from build123d import *

# Parameters (mm, degrees)
SKETCH1_W                = 71.12
SKETCH1_H                = 55.88
PCB_BASE_DEPTH           = 2.54
SKETCH1_4_W              = 78.74
SKETCH1_4_H              = 63.5
SKETCH1_4_W_2            = 71.12
SKETCH1_4_H_2            = 55.88
PCB_WALL_DEPTH           = 25.4
SKETCH2_W                = 27.94
SKETCH2_H                = 15.748
PCB_GAP_DEPTH            = 3.81
LID_HOLE_1_DEPTH         = 3.81
HOLE_SLIDE_1_DEPTH       = 2.54
LID_HOLE_2_START         = -3.81
LID_HOLE_2_DEPTH         = 3.81
HOLE_SLIDE_2_START       = -2.54
HOLE_SLIDE_2_DEPTH       = 2.54
SKETCH5_W                = 27.94
SKETCH5_H                = 5.08
BOSS_EXTRUDE3_DEPTH      = 48.768
BOSS_EXTRUDE4_DEPTH      = 8.89
BOSS_EXTRUDE4_DEPTH_BACK = 1.27
SKETCH7_W                = 38.1
SKETCH7_H                = 25.4
BOSS_EXTRUDE5_DEPTH      = 25.4
SKETCH9_W                = 57.658
SKETCH9_H                = 25.4
BOSS_EXTRUDE6_DEPTH      = 3.81


with BuildPart() as part:
    # Sketch1 → pcb-base (new body)
    with BuildSketch(Plane(origin=(0, 0, 0), x_dir=(1, 0, 0), z_dir=(0, 1, 0))):
        Rectangle(SKETCH1_W, SKETCH1_H)
    extrude(amount=PCB_BASE_DEPTH)

    # Sketch1<4> → pcb-wall (add)
    with BuildSketch(Plane(origin=(0, 0, 0), x_dir=(1, 0, 0), z_dir=(0, 1, 0))):
        Rectangle(SKETCH1_4_W, SKETCH1_4_H)
        Rectangle(SKETCH1_4_W_2, SKETCH1_4_H_2, mode=Mode.SUBTRACT)
    extrude(amount=PCB_WALL_DEPTH)

    # Sketch2 → pcb-gap (cut)
    with BuildSketch(Plane.ZY.offset(39.37)):
        with Locations((-12.7, 12.446)):
            Rectangle(SKETCH2_W, SKETCH2_H)
    extrude(amount=-PCB_GAP_DEPTH, mode=Mode.SUBTRACT)

    # Sketch4 → lid-hole-1 (cut)
    with BuildSketch(Plane(origin=(0, 0, 27.94), x_dir=(-1, 0, 0), z_dir=(0, 0, -1))):
        with BuildLine():
            ThreePointArc((3.175, 17.080851973), (0, 18.415), (-3.175, 17.080851973))
            Line((-3.175, 17.080851973), (-3.175, 13.97))
            Line((-3.175, 13.97), (3.175, 13.97))
            Line((3.175, 13.97), (3.175, 17.080851973))
        make_face()
        with BuildLine():
            Line((-3.175, 13.97), (-3.175, 17.080851973))
            ThreePointArc((-3.175, 17.080851973), (-1.680052083, 9.854729657), (4.445, 13.97))
            ThreePointArc((4.445, 13.97), (4.115270343, 15.650052083), (3.175, 17.080851973))
            Line((3.175, 17.080851973), (3.175, 13.97))
            Line((3.175, 13.97), (-3.175, 13.97))
        make_face()
    extrude(amount=-LID_HOLE_1_DEPTH, mode=Mode.SUBTRACT)

    # Sketch4<6> → hole-slide-1 (cut)
    with BuildSketch(Plane(origin=(0, 0, 27.94), x_dir=(-1, 0, 0), z_dir=(0, 0, -1))):
        with BuildLine():
            Line((3.175, 25.4), (-3.175, 25.4))
            Line((-3.175, 25.4), (-3.175, 17.080851973))
            ThreePointArc((-3.175, 17.080851973), (0, 18.415), (3.175, 17.080851973))
            Line((3.175, 17.080851973), (3.175, 25.4))
        make_face()
    extrude(amount=-HOLE_SLIDE_1_DEPTH, mode=Mode.SUBTRACT)

    # Sketch3 → lid-hole-2 (cut)
    with BuildSketch(Plane.XY.offset(-27.94).offset(LID_HOLE_2_START)):
        with BuildLine():
            Line((-3.175, 17.080851973), (-3.175, 13.97))
            Line((-3.175, 13.97), (3.175, 13.97))
            Line((3.175, 13.97), (3.175, 17.080851973))
            ThreePointArc((3.175, 17.080851973), (0, 18.415), (-3.175, 17.080851973))
        make_face()
        with BuildLine():
            Line((3.175, 13.97), (-3.175, 13.97))
            Line((-3.175, 13.97), (-3.175, 17.080851973))
            ThreePointArc((-3.175, 17.080851973), (-1.680052083, 9.854729657), (4.445, 13.97))
            ThreePointArc((4.445, 13.97), (4.115270343, 15.650052083), (3.175, 17.080851973))
            Line((3.175, 17.080851973), (3.175, 13.97))
        make_face()
    extrude(amount=LID_HOLE_2_DEPTH, mode=Mode.SUBTRACT)

    # Sketch3<5> → hole-slide-2 (cut)
    with BuildSketch(Plane.XY.offset(-27.94).offset(HOLE_SLIDE_2_START)):
        with BuildLine():
            Line((-3.175, 25.4), (-3.175, 17.080851973))
            ThreePointArc((-3.175, 17.080851973), (0, 18.415), (3.175, 17.080851973))
            Line((3.175, 17.080851973), (3.175, 25.4))
            Line((3.175, 25.4), (-3.175, 25.4))
        make_face()
    extrude(amount=HOLE_SLIDE_2_DEPTH, mode=Mode.SUBTRACT)

    # Sketch5 → Boss-Extrude3 (add)
    with BuildSketch(Plane.ZY.offset(39.37)):
        Polygon((-31.75, 25.4), (-31.75, 3.81), (-26.67, 3.81), (-26.67, 4.572), (-26.67, 20.32), (-26.67, 25.4), align=None)
        with Locations((-12.7, 22.86)):
            Rectangle(SKETCH5_W, SKETCH5_H)
        Polygon((1.27, 3.81), (6.35, 3.81), (6.35, 25.4), (1.27, 25.4), (1.27, 20.32), (1.27, 4.572), align=None)
        Polygon((-31.75, 3.81), (-31.75, 0), (6.35, 0), (6.35, 3.81), (1.27, 3.81), (-26.67, 3.81), align=None)
    extrude(amount=BOSS_EXTRUDE3_DEPTH)

    # Sketch7 → Boss-Extrude4 (add, two sides: drawn at the far end of the back side and taken through both)
    with BuildSketch(Plane.ZY.offset(88.138).offset(-BOSS_EXTRUDE4_DEPTH_BACK)):
        with Locations((-12.7, 12.7)):
            Rectangle(SKETCH7_W, SKETCH7_H)
    extrude(amount=BOSS_EXTRUDE4_DEPTH + BOSS_EXTRUDE4_DEPTH_BACK)

    # Sketch8 → Boss-Extrude5 (add)
    with BuildSketch(Plane.XY.offset(6.35)):
        Polygon((-97.028, 25.4), (-97.028, 0), (-39.37, 0), (-39.37, 2.54), (-94.488, 2.54), (-94.488, 22.86), (-39.37, 22.86), (-39.37, 25.4), align=None)
    extrude(amount=BOSS_EXTRUDE5_DEPTH)

    # Sketch9 → Boss-Extrude6 (add)
    with BuildSketch(Plane.XY.offset(31.75)):
        with Locations((-68.199, 12.7)):
            Rectangle(SKETCH9_W, SKETCH9_H)
    extrude(amount=-BOSS_EXTRUDE6_DEPTH)


solid = part.part
Design review of the part built by this model. Coordinates are the model's own, in mm. A direction names the side the tool comes from. Give positions to 0.01 mm unless a question says otherwise; leave off trailing zeros. Loops run counter-clockwise (first coordinate to the right, second up) from the corner with the lowest first, then second, coordinate; pieces in that order, holes last. Notation, with made-up numbers: M -17.5,61.5 L 40.5,61.5 A19 ccw 40.5,80.5 Z; hole C 21,-23.5 d1. An arc over 180 degrees is marked long. One line per question, with ' | ' between items. Start each with the question number.
1. Add section A-A (y = 8). Write out the cut boundary in (x, z), plus the area to 3 significant figures.
2. Add section D-D (z = 17). Write out the cut boundary in (x, y), plus the area to 3 significant figures.
3. For faces 1 (the face through (-58, 25.4, 0)), 2 (the face through (-67, 13, 6.35)), 3 (the face through (-3.175, 21, -29)), list the 3-axis set-ups (+Z, -Z, +X, -X, +Y, -Y) from which the entire face can be reached by the end or side of a thin tool; tool diameter is ignored.
4. Add section C-C (x = -49). Write out the cut boundary in (y, z).
5. The part is to be moulded in two halves that separate along X. For faces 4 (the face through (-97.028, 13, 0)), 5 (the face through (-37, 4.572, -13)), 6 (the face through (-30, 0, 0)), say which applies: released by +X, released by -X, zero draft, split by the parting line, or undercut.
6. To check wall thickness, follow L1, parallel to Z at x = -53, y = 13.5; L2, parallel to Z at x = -86, y = 21.75; L3, parallel to X at y = 24.25, z = 21.5. State the ranges of each line that lie inside material, in increasing order.
7. Insertion check: P1, Ø10, axis at x = 17, z = 15, coming from the -Y side. The pin has a flat end and moves straight along its axis. Give the tip position at first contact, or say it passes through.
8. Add section B-B (z = 3.5). Write out the cut boundary in (x, y), plus the area to 3 significant figures.
Worked out:
1) outline: M -97.03,-31.75 L 39.37,-31.75 L 39.37,31.75 L -97.03,31.75 Z; hole M -94.49,6.35 L -39.37,6.35 L -39.37,27.94 L -94.49,27.94 Z; hole M -86.87,-26.67 L -35.56,-26.67 L -35.56,-27.94 L 35.56,-27.94 L 35.56,27.94 L -35.56,27.94 L -35.56,1.27 L -86.87,1.27 Z | area: 2,060 mm²
2) outline: M -97.03,0 L 39.37,0 L 39.37,25.4 L 35.56,25.4 L 35.56,2.54 L -35.56,2.54 L -35.56,25.4 L -97.03,25.4 Z; hole M -94.49,2.54 L -39.37,2.54 L -39.37,22.86 L -94.49,22.86 Z | area: 719 mm²
3) face 1: +Z, -Z, +X, -X, +Y | face 2: none | face 3: +Y
4) outline: M 0,-31.75 L 25.4,-31.75 L 25.4,31.75 L 0,31.75 Z; hole M 2.54,6.35 L 22.86,6.35 L 22.86,27.94 L 2.54,27.94 Z; hole M 3.81,-26.67 L 20.32,-26.67 L 20.32,1.27 L 3.81,1.27 Z
5) face 4: released by -X | face 5: undercut | face 6: zero draft
6) L1: z = -31.75 to -26.67, 1.27 to 6.35, 27.94 to 31.75 | L2: z = -31.75 to 6.35, 27.94 to 31.75 | L3: x = -97.03 to -35.56, 35.56 to 39.37
7) P1: stops at y = 0
8) outline: M -97.03,0 L 39.37,0 L 39.37,25.4 L 35.56,25.4 L 35.56,2.54 L -35.56,2.54 L -35.56,25.4 L -97.03,25.4 Z | area: 1,840 mm²
